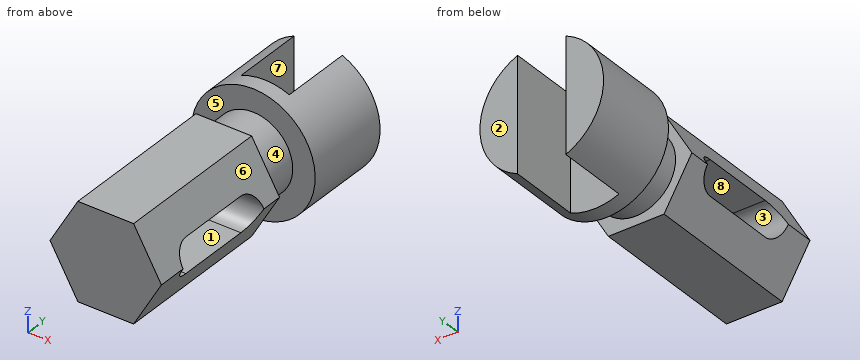
```python
from build123d import *

# Parameters (mm, degrees)
BOSS_EXTRUDE1_DEPTH = 100
SKETCH5_R           = 24.5
BOSS_EXTRUDE3_DEPTH = 25
SKETCH7_R           = 38.461674467
BOSS_EXTRUDE4_DEPTH = 55
SKETCH8_W           = 30
SKETCH8_H           = 78.949061688
CUT_EXTRUDE1_DEPTH  = 45
CUT_EXTRUDE2_DEPTH  = 42.5


with BuildPart() as part:
    # Sketch4 → Boss-Extrude1 (new body)
    with BuildSketch(Plane(origin=(0, 0, 0), x_dir=(1, 0, 0), z_dir=(0, 1, 0))):
        Polygon((34.641016151, 0), (17.320508076, 30), (-17.320508076, 30), (-34.641016151, 0), (-17.320508076, -30), (17.320508076, -30), align=None)
    extrude(amount=BOSS_EXTRUDE1_DEPTH)

    # Sketch5 → Boss-Extrude3 (add)
    with BuildSketch(Plane(origin=(0, 100, 0), x_dir=(1, 0, 0), z_dir=(0, 1, 0))):
        with Locations(Location((0, 0, 0), (0, 0, 270))):
            Circle(SKETCH5_R)
    extrude(amount=BOSS_EXTRUDE3_DEPTH)

    # Sketch7 → Boss-Extrude4 (add)
    with BuildSketch(Plane(origin=(0, 125, 0), x_dir=(1, 0, 0), z_dir=(0, 1, 0))):
        with Locations(Location((0, 0, 0), (0, 0, 270))):
            Circle(SKETCH7_R)
    extrude(amount=BOSS_EXTRUDE4_DEPTH)

    # Sketch8 → Cut-Extrude1 (cut)
    with BuildSketch(Plane(origin=(0, 180, 0), x_dir=(1, 0, 0), z_dir=(0, 1, 0))):
        Rectangle(SKETCH8_W, SKETCH8_H)
    extrude(amount=-CUT_EXTRUDE1_DEPTH, mode=Mode.SUBTRACT)

    # Sketch9 → Cut-Extrude2 (cut, symmetric)
    with BuildSketch(Plane(origin=(0, 0, 0), x_dir=(0, 0, -1), z_dir=(1, 0, 0))):
        with BuildLine():
            Line((10.959896638, 75.869076848), (10.959896638, 29.285757766))
            ThreePointArc((10.959896638, 29.285757766), (0, 18.325861128), (-10.959896638, 29.285757766))
            Line((-10.959896638, 29.285757766), (-10.959896638, 75.869076848))
            ThreePointArc((-10.959896638, 75.869076848), (0, 86.828973486), (10.959896638, 75.869076848))
        make_face()
    extrude(amount=CUT_EXTRUDE2_DEPTH, both=True, mode=Mode.SUBTRACT)


solid = part.part
```
Input: part model. Units: mm. Frame: model coordinates. Face numbers are marked on the shaded views. A direction names the side the tool comes from. Coordinates: 2 decimals unless noted, no trailing zeros. Loops run counter-clockwise (first coordinate to the right, second up) from the corner with the lowest first, then second, coordinate; pieces in that order, holes last. Notation, with made-up numbers: (50, -7.5) -> (61, -7.5) arc R31 ccw to (61, 30.5) -> close; hole circle Ø3 at (87.25, -39). An arc over 180 degrees is marked (long way). Use a Markdown table: item, result.
1) Pull-direction query (Z, two-part tool) for the marked faces 1, 2, 3 and 4; classes: released by +Z, released by -Z, zero draft, split by the parting line, or undercut.
Results found:
| item | result |
|---|---|
| face 1 | undercut |
| face 2 | zero draft |
| face 3 | undercut |
| face 4 | split by the parting line |
2) Material intervals for line 1 along Y through (x, z) = (21.5, -16); line 2 along Z through (x, y) = (4.5, 39); line 3 along Y through (x, z) = (-1.5, 29), sorted ascending. Write a range as from..to.
Results found:
| item | result |
|---|---|
| line 1 | y = 0..100, 125..180 |
| line 2 | z = -30..-10.96, 10.96..30 |
| line 3 | y = 0..100, 125..135 |
3) Contact query for flat-ended pins moving along their axis: pin 1 (6 mm diameter, centred on x = -29, y = 46.5, fed in from -Z); pin 2 (4 mm diameter, centred on x = -3.5, y = 82.5, fed in from -Z); pin 3 (6 mm diameter, centred on x = -25, y = 153.5, fed in from +Z). Output: stop coordinate, or through.
Results found:
| item | result |
|---|---|
| pin 1 | stops at z = -14.97 |
| pin 2 | stops at z = -30 |
| pin 3 | stops at z = 31.55 |
4) Cut plane C-C (z = -2). Return the cut outline in (x, y), then the cut area to 3 significant figures.
Results found:
| item | result |
|---|---|
| outline | (-38.41, 125) -> (-24.42, 125) -> (-24.42, 100) -> (-33.49, 100) -> (-33.49, 86.64) -> (33.49, 86.64) -> (33.49, 100) -> (24.42, 100) -> (24.42, 125) -> (38.41, 125) -> (38.41, 180) -> (15, 180) -> (15, 135) -> (-15, 135) -> (-15, 180) -> (-38.41, 180) -> close; (-33.49, 0) -> (33.49, 0) -> (33.49, 18.51) -> (-33.49, 18.51) -> close |
| area | 6,230 mm2 |
5) Cut plane D-D (z = -21). Return the cut outline in (x, y), then the cut area to 3 significant figures.
Results found:
| item | result |
|---|---|
| outline | (-32.22, 125) -> (-12.62, 125) -> (-12.62, 100) -> (-22.52, 100) -> (-22.52, 0) -> (22.52, 0) -> (22.52, 100) -> (12.62, 100) -> (12.62, 125) -> (32.22, 125) -> (32.22, 180) -> (15, 180) -> (15, 135) -> (-15, 135) -> (-15, 180) -> (-32.22, 180) -> close |
| area | 7,330 mm2 |
6) Cut plane A-A (x = 0). Return the cut outline in (y, z).
Results found:
| item | result |
|---|---|
| outline | (0, -30) -> (100, -30) -> (100, -24.5) -> (125, -24.5) -> (125, -38.46) -> (135, -38.46) -> (135, 38.46) -> (125, 38.46) -> (125, 24.5) -> (100, 24.5) -> (100, 30) -> (0, 30) -> close; hole (29.29, -10.96) -> (75.87, -10.96) arc R10.96 ccw to (75.87, 10.96) -> (29.29, 10.96) arc R10.96 ccw to start |
7) Cut plane B-B (y = 51). Return the cut outline in (x, z), then the cut area to 3 significant figures.
Results found:
| item | result |
|---|---|
| outline | (-28.31, -10.96) -> (-17.32, -30) -> (17.32, -30) -> (28.31, -10.96) -> close; (-28.31, 10.96) -> (28.31, 10.96) -> (17.32, 30) -> (-17.32, 30) -> close |
| area | 1,740 mm2 |
8) Access query for the marked faces 5, 6, 7 and 8. Directions: +Z, -Z, +X, -X, +Y, -Y. A direction counts if a zero-diameter tool reaches every point of the face in a straight line with its end or side. Return the directions, or none.
Results found:
| item | result |
|---|---|
| face 5 | none |
| face 6 | +Z, +X, -Y |
| face 7 | +Z, -Z, +Y |
| face 8 | +X, -X |
